```python
from build123d import *

# Parameters (mm, degrees)
SKETCH_1_W          = 64
SKETCH_1_H          = 64
SKETCH_1_R          = 23.5
EXTRUDE_1_DEPTH     = 2.5
SKETCH_2_W          = 64
SKETCH_2_H          = 64
SKETCH_2_R          = 25.1
EXTRUDE_2_DEPTH     = 7.5
SKETCH_3_R          = 2.1
CUT_EXTRUDE_1_DEPTH = 20
FILLET_1_R          = 10


with BuildPart() as part:
    # 草图1 → 凸台-拉伸1 (new body)
    with BuildSketch(Plane(origin=(0, 0, 0), x_dir=(1, 0, 0), z_dir=(0, 1, 0))):
        Rectangle(SKETCH_1_W, SKETCH_1_H)
        with Locations(Location((0, 0, 0), (0, 0, 270))):
            Circle(SKETCH_1_R, mode=Mode.SUBTRACT)
    extrude(amount=EXTRUDE_1_DEPTH)

    # 草图2 → 凸台-拉伸2 (add)
    with BuildSketch(Plane(origin=(0, 2.5, 0), x_dir=(1, 0, 0), z_dir=(0, 1, 0))):
        Rectangle(SKETCH_2_W, SKETCH_2_H)
        with Locations(Location((0, 0, 0), (0, 0, 270))):
            Circle(SKETCH_2_R, mode=Mode.SUBTRACT)
    extrude(amount=EXTRUDE_2_DEPTH)

    # 草图3 → 切除-拉伸1 (cut)
    with BuildSketch(Plane(origin=(0, 10, 0), x_dir=(1, 0, 0), z_dir=(0, 1, 0))):
        with Locations(Location((24.04163056, 24.04163056, 0), (0, 0, 270))):
            Circle(SKETCH_3_R)
        with Locations(Location((24.04163056, -24.04163056, 0), (0, 0, 270))):
            Circle(SKETCH_3_R)
        with Locations(Location((-24.04163056, -24.04163056, 0), (0, 0, 270))):
            Circle(SKETCH_3_R)
        with Locations(Location((-24.04163056, 24.04163056, 0), (0, 0, 270))):
            Circle(SKETCH_3_R)
    extrude(amount=-CUT_EXTRUDE_1_DEPTH, mode=Mode.SUBTRACT)

    # 圆角1
    fillet_1_edges = [part.edges().sort_by_distance(p)[0] for p in [
        (32, 5, 32),
        (-32, 5, 32),
        (-32, 5, -32),
        (32, 5, -32),
    ]]
    fillet(fillet_1_edges, radius=FILLET_1_R)


solid = part.part
```
Model file for the job. Use its own axes, mm. A direction names the side the tool comes from. Give positions to 0.01 mm unless a question says otherwise; leave off trailing zeros. Loops run counter-clockwise (first coordinate to the right, second up) from the corner with the lowest first, then second, coordinate; pieces in that order, holes last. Notation, with made-up numbers: (73, -17.5) -> (107, -17.5) arc R36 cw to (107, 19.5) -> close; hole circle Ø9 at (-34, -39). An arc over 180 degrees is marked (long way). Use CSV: the item, a comma, the result in double quotes. Start each with the question number.
1) Tool access for faces 4 (the flat face through (-7.6, 2.5, -22.4)), 5 (the flat face through (0, 5, 32)): list every direction of +Z, -Z, +X, -X, +Y, -Y with a clear straight run to the whole face (end or side of a thin tool).
2) Slice it at C-C on y = 3.5. Give the cut face in (x, z), plus the area to 3 significant figures.
3) Flat gauge pin, fed straight in: pin 1 Ø1.5 at (x, z) = (-18.5, 20) entering from -Y. Where does the tip first touch, or does it go through?
4) Wall check: line 1 (X direction, y = 2.25, z = -24.5); line 2 (X direction, y = 9.5, z = -17); line 3 (Z direction, x = -5.5, y = 5.25). Give the ranges that are in metal, low to high.
5) Slice it at B-B on z = 0. Give the cut face in (x, y), plus the area to 3 significant figures.
6) Slice it at D-D on x = 27. Give the cut face in (y, z).
7) Mould opens along X. For faces 1 (the cylindrical face through (23.24, 5.07, -22.1)), 2 (the flat face through (-22, 10, -15)), 3 (the cylindrical face through (-29.15, 5.07, 28.99)) say: released by +X, released by -X, zero draft, split by the parting line, or undercut.
8) Slice it at A-A on x = 0. Give the cut face in (y, z).
Computed values:
1,face 4,"+Y"
1,face 5,"+Z, +X, -X, +Y, -Y"
2,outline,"(-32, -22) arc R10 ccw to (-22, -32) -> (22, -32) arc R10 ccw to (32, -22) -> (32, 22) arc R10 ccw to (22, 32) -> (-22, 32) arc R10 ccw to (-32, 22) -> close; hole circle Ø4.2 at (-24.04, -24.04); hole circle Ø4.2 at (-24.04, 24.04); hole circle Ø50.2 at (0, 0); hole circle Ø4.2 at (24.04, -24.04); hole circle Ø4.2 at (24.04, 24.04)"
2,area,"1,980 mm^2"
3,pin 1,"stops at y = 0"
4,line 1,"x = -31.68 to -26.09, -21.99 to 21.99, 26.09 to 31.68"
4,line 2,"x = -32 to -18.47, 18.47 to 32"
4,line 3,"z = -32 to -24.49, 24.49 to 32"
5,outline,"(-32, 0) -> (-23.5, 0) -> (-23.5, 2.5) -> (-25.1, 2.5) -> (-25.1, 10) -> (-32, 10) -> close; (23.5, 0) -> (32, 0) -> (32, 10) -> (25.1, 10) -> (25.1, 2.5) -> (23.5, 2.5) -> close"
5,area,"146 mm^2"
6,outline,"(0, -30.66) -> (10, -30.66) -> (10, 30.66) -> (0, 30.66) -> close"
7,face 1,"undercut"
7,face 2,"zero draft"
7,face 3,"released by -X"
8,outline,"(0, -32) -> (10, -32) -> (10, -25.1) -> (2.5, -25.1) -> (2.5, -23.5) -> (0, -23.5) -> close; (0, 23.5) -> (2.5, 23.5) -> (2.5, 25.1) -> (10, 25.1) -> (10, 32) -> (0, 32) -> close"
